Design review of the part built by this model. Coordinates are the model's own, in mm. Face numbers are marked on the shaded views. A direction names the side the tool comes from. Give positions to 0.01 mm unless a question says otherwise; leave off trailing zeros. Loops run counter-clockwise (first coordinate to the right, second up) from the corner with the lowest first, then second, coordinate; pieces in that order, holes last. Notation, with made-up numbers: M 63,32 L 87,32 A16 ccw 87,48 Z; hole C -25,4 d11. An arc over 180 degrees is marked long. Use a Markdown table: item, result. Add a question column.
(1) For the marked faces 3 and 4, list the 3-axis set-ups (+Z, -Z, +X, -X, +Y, -Y) from which the entire face can be reached by the end or side of a thin tool; tool diameter is ignored.
(2) For probe 1 along Y at (x, z) = (1, 0); probe 2 along Z at (x, y) = (9, 12); probe 3 along Y at (x, z) = (1.5, 0), list the stretches that pass through material, from the lowest coordinate up.
(3) Draft analysis for pull direction Z (two halves, no side actions). For the marked faces 1 and 2, state which applies: pulls with the +Z half, pulls with the -Z half, needs draft (parallel to the pull), parting line crosses it, or undercut.
(4) Add section C-C, the plane x = 2. Give the boundary of the cut face in (y, z) (1 decimal), then the cut area to 3 significant figures.
(5) Insertion check: pin 1 Ø10 at (y, z) = (45.5, -5) entering from +X; pin 2 Ø3 at (x, y) = (1.5, 50.5) entering from +Z; pin 3 Ø1.5 at (x, y) = (-1.5, 12) entering from -Z. Each pin has a flat end and moves straight along its axis. Give the tip position at first contact, or say it passes through.
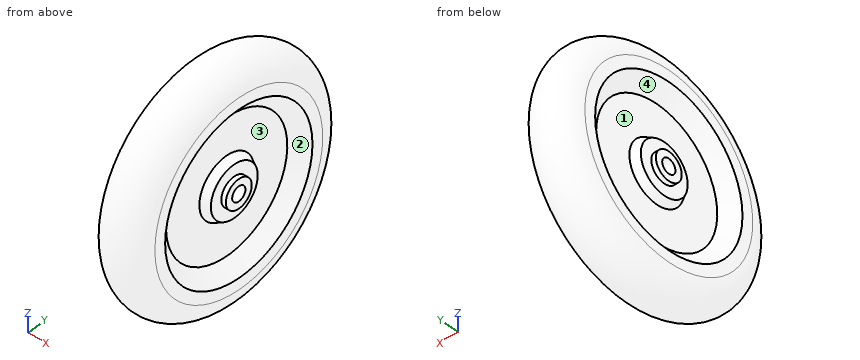
```python
from build123d import *


with BuildPart() as part:
    # Sketch1 → Revolve1 (revolve)
    with BuildSketch(Plane.XY, mode=Mode.PRIVATE) as revolve1_sk:
        with BuildLine():
            Line((-15.875, 4.7625), (15.875, 4.7625))
            Line((15.875, 4.7625), (15.875, 9.311015131))
            Line((15.875, 9.311015131), (12.83850319, 9.311015131))
            Line((12.83850319, 9.311015131), (12.83850319, 16.850886509))
            Line((12.83850319, 16.850886509), (7.782087298, 19.62375974))
            Line((7.782087298, 19.62375974), (7.782087298, 43.587197627))
            Line((7.782087298, 43.587197627), (15.875, 52.96008786))
            Line((15.875, 52.96008786), (15.875, 60.325))
            ThreePointArc((15.875, 60.325), (0, 76.2), (-15.875, 60.325))
            Line((-15.875, 60.325), (-15.875, 52.96008786))
            Line((-15.875, 52.96008786), (-7.782087298, 43.587197627))
            Line((-7.782087298, 43.587197627), (-7.782087298, 19.62375974))
            Line((-7.782087298, 19.62375974), (-12.83850319, 16.850886509))
            Line((-12.83850319, 16.850886509), (-12.83850319, 9.311015131))
            Line((-12.83850319, 9.311015131), (-15.875, 9.311015131))
            Line((-15.875, 9.311015131), (-15.875, 4.7625))
        make_face()
    revolve(revolve1_sk.sketch.rotate(Axis((-1000, 0, 0), (1, 0, 0)), 90), axis=Axis((-1000, 0, 0), (1, 0, 0)))


solid = part.part
```
Established:
| question | item | result |
|---|---|---|
| 1 | face 3 | +X |
| 1 | face 4 | -X |
| 2 | probe 1 | -76.17 to -4.76, 4.76 to 76.17 |
| 2 | probe 2 | -72.41 to -43.37, -14.67 to 14.67, 43.37 to 72.41 |
| 2 | probe 3 | -76.13 to -4.76, 4.76 to 76.13 |
| 3 | face 1 | undercut |
| 3 | face 2 | undercut |
| 4 | outline | C 0,0 d152.1; hole C 0,0 d9.5 |
| 4 | area | 18,100 mm^2 |
| 5 | pin 1 | x = 13.99 |
| 5 | pin 2 | z = 58.28 |
| 5 | pin 3 | z = -75.31 |
